Autodesk Inventor part; units mm, degrees
ref_plane "YZ Plane" through (0, 0, 0) normal (1, 0, 0) x (0, 1, 0)
ref_plane "XZ Plane" through (0, 0, 0) normal (0, 1, 0) x (-1, 0, 0)
ref_plane "XY Plane" through (0, 0, 0) normal (0, 0, 1) x (1, 0, 0)
sketch "Sketch1" plane through (0, 0, 0) normal (0, 0, 1) x (1, 0, 0)
  line L0 (-152.4, -101.6) -> (152.4, -101.6)
  line L1 (152.4, -101.6) -> (152.4, 101.6)
  line L2 (152.4, 101.6) -> (-152.4, 101.6)
  line L3 (-152.4, 101.6) -> (-152.4, -101.6)
  line L4 (-152.4, -101.6) -> (152.4, 101.6) construction
  line L5 (152.4, -101.6) -> (-152.4, 101.6) construction
  line L6 (152.4, 101.6) -> (152.4, 228.6)
  line L7 (152.4, 228.6) -> (457.2, 0)
  line L8 (457.2, 0) -> (152.4, -228.6)
  line L9 (152.4, -228.6) -> (152.4, -101.6)
  point P0 (0, 0)
  dimension "d0" = 304.8
  dimension "d1" = 203.2
  dimension "d2" = 304.8
  dimension "d3" = 457.2
extrude "Extrusion1" add sketch "Sketch1" along normal mid plane 50.8
properties part number "AirFlow"
Check sheet for the modelled part. Datum: model origin and axes. Units: mm. A direction names the side the tool comes from. Give positions to 0.01 mm unless a question says otherwise; leave off trailing zeros. Order: outer loops, then holes, each group sorted by start corner. A loop starts at its lowest first (then second) coordinate and runs counter-clockwise, first axis right, second up. Notation, with made-up numbers: M 84.5,27 L 122.5,27 A19 ccw 122.5,37 Z; hole C -1.75,24.25 d10. An arc over 180 degrees is marked long. Answer in a Markdown table with one row per item.
1) Access from +Z, -Z, +X, -X, +Y, -Y to the whole of each face (thin tool, end or side, straight path). Record for faces 1 (the flat face through (148, 3, 25.4)), 2 (the flat face through (152.4, 164, 0)), 3 (the flat face through (152.4, -166, 0)).
Filled sheet:
| item | result |
|---|---|
| face 1 | +Z, +X, -X, +Y, -Y |
| face 2 | +Z, -Z, -X, +Y |
| face 3 | +Z, -Z, -X, -Y |
2) Gauge pin test, flat ends, axial feed: P1, Ø6, axis at x = -7.5, z = -17.5, coming from the -Y side; P2, Ø10, axis at x = 231, z = 9, coming from the -Y side; P3, Ø5, axis at y = 56, z = -20, coming from the +X side. Record the tip position at first contact, or that the pin passes through.
Filled sheet:
| item | result |
|---|---|
| P1 | stops at y = -101.6 |
| P2 | stops at y = -173.4 |
| P3 | stops at x = 385.87 |
3) Cross-section at C-C, the plane x = 297. Enter the section's corners in (y, z).
Filled sheet:
| item | result |
|---|---|
| outline | M -120.15,-25.4 L 120.15,-25.4 L 120.15,25.4 L -120.15,25.4 Z |
4) Cross-section at B-B, the plane y = -201. Enter the section's corners in (x, z).
Filled sheet:
| item | result |
|---|---|
| outline | M 152.4,-25.4 L 189.2,-25.4 L 189.2,25.4 L 152.4,25.4 Z |
5) Thickness scan on L1, parallel to Y at x = 15, z = 10.5; L2, parallel to Y at x = 220.5, z = -21 (3 decimals); L3, parallel to X at y = 148, z = 6.5. Record the ranges inside material, lowest first. Write a range as [from, to].
Filled sheet:
| item | result |
|---|---|
| L1 | y = [-101.6, 101.6] |
| L2 | y = [-177.525, 177.525] |
| L3 | x = [152.4, 259.87] |
6) Cross-section at A-A, the plane z = -11. Enter the section's corners in (x, y).
Filled sheet:
| item | result |
|---|---|
| outline | M -152.4,-101.6 L 152.4,-101.6 L 152.4,-228.6 L 457.2,0 L 152.4,228.6 L 152.4,101.6 L -152.4,101.6 Z |
